Input: part model. Units: mm. Frame: model coordinates. A direction names the side the tool comes from. Give positions to 0.01 mm unless a question says otherwise; leave off trailing zeros. Loops run counter-clockwise (first coordinate to the right, second up) from the corner with the lowest first, then second, coordinate; pieces in that order, holes last. Notation, with made-up numbers: M 35.5,58 L 94.5,58 A28 ccw 94.5,90 Z; hole C 2.5,-38.75 d1. An arc over 180 degrees is marked long. One line per item, written item: value. Start each with the question number.
(1) Pin query (flat end, axial travel): P1, Ø0.6, axis at y = 11.5, z = -21.5, coming from the -X side; P2, Ø4.5, axis at x = -13.5, y = 11.5, coming from the +Z side; P3, Ø10.5, axis at x = -23.5, y = 18, coming from the -Z side; P4, Ø5, axis at x = -2, y = 13.5, coming from the +Z side. Return the tip coordinate at first contact, or that it passes through.
(2) Ray query, line 1 along X through (y, z) = (10.5, 61); line 2 along Z through (x, y) = (-23, 13.5); line 3 along X through (y, z) = (20, -17). Return the intervals inside material, ascending. Write a range as from..to.
(3) Section A-A on z = 50. Output: boundary loops of the cut face in (x, y), plus the area to 3 significant figures.
(4) Section B-B on z = 25.5. Output: boundary loops of the cut face in (x, y), plus the area to 3 significant figures.
(5) Pull-direction query (Z, two-part tool) for faces 1 (the flat face through (0, 9, -72.5)), 2 (the flat face through (-25, 25, -2.5)), 3 (the flat face through (8, 36, 37)), 4 (the flat face through (20.249, 11, -52)); classes: released by +Z, released by -Z, zero draft, split by the parting line, or undercut.
(6) Section C-C on z = -24.5. Output: boundary loops of the cut face in (x, y), plus the area to 3 significant figures.
(7) Access query for faces 5 (the flat face through (6.87, 7.48, -32.08)), 6 (the flat face through (-20.25, 30, -23)), 7 (the flat face through (7, 36, 63)), 8 (the flat face through (-3.75, 16, -32)). Directions: +Z, -Z, +X, -X, +Y, -Y. A direction counts if a zero-diameter tool reaches every point of the face in a straight line with its end or side. Return the directions, or none.
```python
from build123d import *

# Parameters (mm, degrees)
SKETCH_1_W                = 100
SKETCH_1_H                = 185
EXTRUDE_1_DEPTH           = 100
SKETCH_2_W                = 100
SKETCH_2_H                = 3.8
CUT_EXTRUDE_1_DEPTH       = 155
CUT_EXTRUDE_2_DEPTH       = 155
SKETCH_4_W                = 25.5
SKETCH_4_H                = 25.5
CUT_EXTRUDE_3_DEPTH       = 79
SKETCH_6_W                = 89.706259743
SKETCH_6_H                = 10
SKETCH_6_W_2              = 10.293740257
CUT_EXTRUDE_4_DEPTH       = 146.107718609
CUT_EXTRUDE_5_DEPTH       = 169.985946161
CUT_EXTRUDE_5_DEPTH_BACK  = 169.985946161
SKETCH_7_W                = 20
SKETCH_7_H                = 3.8
EXTRUDE_4_DEPTH           = 160
SKETCH_10_W               = 16
SKETCH_10_H               = 1.8
CUT_EXTRUDE_6_DEPTH       = 155
SKETCH_13_W               = 20
SKETCH_13_H               = 175
CUT_EXTRUDE_7_DEPTH       = 143.515578096
SKETCH_14_W               = 175
SKETCH_14_H               = 50
CUT_EXTRUDE_8_DEPTH       = 149.849756466
SKETCH_15_W               = 60
SKETCH_15_H               = 10
CUT_EXTRUDE_9_DEPTH       = 108.660066877
SKETCH_16_W               = 60
SKETCH_16_H               = 14.5
CUT_EXTRUDE_10_DEPTH      = 108.660066877
CUT_EXTRUDE_11_DEPTH      = 111.381157812
CUT_EXTRUDE_21_DEPTH      = 162.400898529
CUT_EXTRUDE_21_DEPTH_BACK = 140.5
CUT_EXTRUDE_26_DEPTH      = 111.381157983
SKETCH_34_W               = 10
SKETCH_34_H               = 20
CUT_EXTRUDE_31_DEPTH      = 96.490523251
SKETCH_35_W               = 18.74373947
SKETCH_35_H               = 80.5
CUT_EXTRUDE_32_DEPTH      = 14
CUT_EXTRUDE_35_DEPTH      = 60
CUT_EXTRUDE_36_DEPTH      = 140.5
SKETCH_43_W               = 0.25
SKETCH_43_H               = 0.002112168
CUT_EXTRUDE_37_DEPTH      = 140.5
SKETCH_44_W               = 7.5
SKETCH_44_H               = 0.502112168
CUT_EXTRUDE_38_DEPTH      = 80.4999
SKETCH_45_W               = 9.75
SKETCH_45_H               = 20
SKETCH_45_W_2             = 9.75146362
CUT_EXTRUDE_39_DEPTH      = 96.490523251
SKETCH_46_W               = 0.24853638
SKETCH_46_H               = 20
SKETCH_46_W_2             = 0.25
EXTRUDE_5_DEPTH           = 31.697888
CUT_EXTRUDE_40_DEPTH      = 106.399537724
CUT_EXTRUDE_40_DEPTH_BACK = 106.399537724
SKETCH_54_W               = 25.5
SKETCH_54_H               = 0.5
CUT_EXTRUDE_41_DEPTH      = 29


with BuildPart() as part:
    # 草图1 → 凸台-拉伸1 (new body)
    with BuildSketch(Plane(origin=(0, 0, 0), x_dir=(1, 0, 0), z_dir=(0, 1, 0))):
        Rectangle(SKETCH_1_W, SKETCH_1_H)
    extrude(amount=EXTRUDE_1_DEPTH)

    # 草图2 → 切除-拉伸1 (cut)
    with BuildSketch(Plane.XY.offset(92.5)):
        with Locations((0, 1.9)):
            Rectangle(SKETCH_2_W, SKETCH_2_H)
    extrude(amount=-CUT_EXTRUDE_1_DEPTH, mode=Mode.SUBTRACT)

    # 草图3 → 切除-拉伸2 (cut)
    with BuildSketch(Plane.XY.offset(92.5)):
        with BuildLine():
            Line((-20, 3.8), (-3.51, 3.8))
            ThreePointArc((-3.51, 3.8), (-3.949598778, 3.901619975), (-4.3, 4.185860522))
            Line((-4.3, 4.185860522), (-9.371869735, 10.69267521))
            ThreePointArc((-9.371869735, 10.69267521), (-9.267749528, 11.143089764), (-8.9765156, 11.502112168))
            Line((-8.9765156, 11.502112168), (-4.5, 11.502112168))
            ThreePointArc((-4.5, 11.502112168), (-4.146446609, 11.648558777), (-4, 12.002112168))
            Line((-4, 12.002112168), (-4, 16.002112168))
            Line((-4, 16.002112168), (-20, 16.002112168))
            Line((-20, 16.002112168), (-20, 3.8))
        make_face()
        with BuildLine():
            ThreePointArc((4.3, 4.185860522), (3.949598778, 3.901619975), (3.51, 3.8))
            Line((3.51, 3.8), (20, 3.8))
            Line((20, 3.8), (20, 16.002112168))
            Line((20, 16.002112168), (4, 16.002112168))
            Line((4, 16.002112168), (4, 12.002112168))
            ThreePointArc((4, 12.002112168), (4.146446609, 11.648558777), (4.5, 11.502112168))
            Line((4.5, 11.502112168), (8.9765156, 11.502112168))
            ThreePointArc((8.9765156, 11.502112168), (9.426930154, 11.220838522), (9.371869735, 10.69267521))
            Line((9.371869735, 10.69267521), (4.3, 4.185860522))
        make_face()
    extrude(amount=-CUT_EXTRUDE_2_DEPTH, mode=Mode.SUBTRACT)

    # 草图4 → 切除-拉伸3 (cut)
    with BuildSketch(Plane(origin=(0, 100, 0), x_dir=(1, 0, 0), z_dir=(0, 1, 0))):
        with Locations((7.75, -50.25)):
            Rectangle(SKETCH_4_W, SKETCH_4_H)
    extrude(amount=-CUT_EXTRUDE_3_DEPTH, mode=Mode.SUBTRACT)

    # 草图6 → 切除-拉伸4 (cut, through all)
    with BuildSketch(Plane(origin=(0, 100, 0), x_dir=(1, 0, 0), z_dir=(0, 1, 0))):
        with Locations((5.146870128, 87.5)):
            Rectangle(SKETCH_6_W, SKETCH_6_H)
        with Locations((-44.853129872, 87.5)):
            Rectangle(SKETCH_6_W_2, SKETCH_6_H)
    extrude(amount=-CUT_EXTRUDE_4_DEPTH, mode=Mode.SUBTRACT)

    # 草图7 → 切除-拉伸5 (cut, two sides: drawn at the far end of the back side and taken through both)
    with BuildSketch(Plane.ZY.offset(50).offset(-CUT_EXTRUDE_5_DEPTH_BACK)):
        with Locations((-72.5, 1.9)):
            Rectangle(SKETCH_7_W, SKETCH_7_H)
    extrude(amount=CUT_EXTRUDE_5_DEPTH + CUT_EXTRUDE_5_DEPTH_BACK, mode=Mode.SUBTRACT)

    # 草图9 → 凸台-拉伸4 (add)
    with BuildSketch(Plane.XY.offset(92.5)):
        Polygon((-9.371869735, 10.69267521), (-9.371869735, 13.29267521), (-4, 13.29267521), (4, 13.29267521), (9.371869735, 13.29267521), (9.371869735, 10.69267521), align=None)
    extrude(amount=-EXTRUDE_4_DEPTH)

    # 草图10 → 切除-拉伸6 (cut)
    with BuildSketch(Plane.XY.offset(92.5)):
        with Locations((-12, 16.902112168)):
            Rectangle(SKETCH_10_W, SKETCH_10_H)
        Polygon((4, 16.002112168), (4, 17.802112168), (19.99853638, 17.802112168), (20, 16.002112168), align=None)
    extrude(amount=-CUT_EXTRUDE_6_DEPTH, mode=Mode.SUBTRACT)

    # 草图13 → 切除-拉伸7 (cut, through all)
    with BuildSketch(Plane.XZ.offset(-3.8)):
        with Locations((-40, 5)):
            Rectangle(SKETCH_13_W, SKETCH_13_H)
        with Locations((40, 5)):
            Rectangle(SKETCH_13_W, SKETCH_13_H)
    extrude(amount=-CUT_EXTRUDE_7_DEPTH, mode=Mode.SUBTRACT)

    # 草图14 → 切除-拉伸8 (cut, through all)
    with BuildSketch(Plane(origin=(30, 0, 0), x_dir=(0, 0, -1), z_dir=(1, 0, 0))):
        with Locations((-5, 75)):
            Rectangle(SKETCH_14_W, SKETCH_14_H)
    extrude(amount=-CUT_EXTRUDE_8_DEPTH, mode=Mode.SUBTRACT)

    # 草图15 → 切除-拉伸9 (cut, through all)
    with BuildSketch(Plane.XZ.offset(-3.8)):
        with Locations((0, -77.5)):
            Rectangle(SKETCH_15_W, SKETCH_15_H)
    extrude(amount=-CUT_EXTRUDE_9_DEPTH, mode=Mode.SUBTRACT)

    # 草图16 → 切除-拉伸10 (cut, through all)
    with BuildSketch(Plane(origin=(0, 50, 0), x_dir=(1, 0, 0), z_dir=(0, 1, 0))):
        with Locations((0, -85.25)):
            Rectangle(SKETCH_16_W, SKETCH_16_H)
    extrude(amount=-CUT_EXTRUDE_10_DEPTH, mode=Mode.SUBTRACT)

    # 草图17 → 切除-拉伸11 (cut, through all)
    with BuildSketch(Plane(origin=(30, 0, 0), x_dir=(0, 0, -1), z_dir=(1, 0, 0))):
        with BuildLine():
            Line((72.5, 50), (-22.5, 50))
            add(Edge.make_bspline(
                [(-22.5, 50), (-9.330669895, 49.706144403), (11.085821801, 46.827148239), (38.239751221, 39.498978447), (59.688603115, 33.272875951), (70.679662454, 22.295526596), (72.5, 15.311284203)],
                knots=[0, 0, 0, 0, 0.374533404, 0.581855131, 0.802431491, 1, 1, 1, 1], degree=3))
            Line((72.5, 15.311284203), (72.5, 50))
        make_face()
    extrude(amount=-CUT_EXTRUDE_11_DEPTH, mode=Mode.SUBTRACT)

    # 草图24 → 切除-拉伸21 (cut, two sides: drawn at the far end of the back side and taken through both)
    with BuildSketch(Plane.XY.offset(78).offset(-CUT_EXTRUDE_21_DEPTH_BACK)):
        with BuildLine():
            Line((9.371869735, 11.309008937), (9.371869735, 10.69267521))
            ThreePointArc((9.371869735, 10.69267521), (9.477785695, 11.000842073), (9.371869735, 11.309008937))
        make_face()
    extrude(amount=CUT_EXTRUDE_21_DEPTH + CUT_EXTRUDE_21_DEPTH_BACK, mode=Mode.SUBTRACT)

    # 草图28 → 切除-拉伸26 (cut, through all)
    with BuildSketch(Plane(origin=(30, 0, 0), x_dir=(0, 0, -1), z_dir=(1, 0, 0))):
        with BuildLine():
            Line((-70.5, 50), (-78, 50))
            Line((-78, 50), (-78, 31.982866201))
            add(Edge.make_bspline(
                [(-70.5, 50), (-78.410932033, 48.656434308), (-77.0737544, 36.843285786), (-78, 31.982866201)],
                knots=[0, 0, 0, 0, 1, 1, 1, 1], degree=3))
        make_face()
    extrude(amount=-CUT_EXTRUDE_26_DEPTH, mode=Mode.SUBTRACT)

    # 草图34 → 切除-拉伸31 (cut, through all)
    with BuildSketch(Plane.XZ.offset(-3.8)):
        with Locations((-25, -32.5)):
            Rectangle(SKETCH_34_W, SKETCH_34_H)
        with Locations((25, -32.5)):
            Rectangle(SKETCH_34_W, SKETCH_34_H)
    extrude(amount=-CUT_EXTRUDE_31_DEPTH, mode=Mode.SUBTRACT)

    # 草图35 → 切除-拉伸32 (cut)
    with BuildSketch(Plane.XZ.offset(-3.8)):
        with Locations((0, 37.75)):
            Rectangle(SKETCH_35_W, SKETCH_35_H)
    extrude(amount=-CUT_EXTRUDE_32_DEPTH, mode=Mode.SUBTRACT)

    # 草图40 → 切除-拉伸35 (cut)
    with BuildSketch(Plane.XY.offset(-2.5)):
        Polygon((4, 13.29267521), (4, 17.8), (3.75, 17.8), (3.75, 12.79267521), (9.371869735, 12.79267521), (9.371869735, 13.29267521), align=None)
        Polygon((-3.75, 17.8), (-4, 17.8), (-4, 13.29267521), (-9.371869735, 13.29267521), (-9.371869735, 12.79267521), (-3.75, 12.79267521), align=None)
    extrude(amount=-CUT_EXTRUDE_35_DEPTH, mode=Mode.SUBTRACT)

    # 草图41 → 切除-拉伸36 (cut)
    with BuildSketch(Plane.XY.offset(78)):
        Polygon((-3.75, 18.302112168), (-20.25, 18.302112168), (-20.25, 3.8), (-20, 3.8), (-20, 17.802112168), (-3.75, 17.802112168), align=None)
        Polygon((3.75, 18.302112168), (3.75, 17.802112168), (19.99853638, 17.802112168), (19.99853638, 3.8), (20.24853638, 3.8), (20.24853638, 18.302112168), align=None)
    extrude(amount=-CUT_EXTRUDE_36_DEPTH, mode=Mode.SUBTRACT)

    # 草图43 → 切除-拉伸37 (cut)
    with BuildSketch(Plane.XY.offset(78)):
        with Locations((-3.875, 17.801056084)):
            Rectangle(SKETCH_43_W, SKETCH_43_H)
        with Locations((3.875, 17.801056084)):
            Rectangle(SKETCH_43_W, SKETCH_43_H)
    extrude(amount=-CUT_EXTRUDE_37_DEPTH, mode=Mode.SUBTRACT)

    # 草图44 → 切除-拉伸38 (cut)
    with BuildSketch(Plane.XY.offset(78)):
        with Locations((0, 18.051056084)):
            Rectangle(SKETCH_44_W, SKETCH_44_H)
    extrude(amount=-CUT_EXTRUDE_38_DEPTH, mode=Mode.SUBTRACT)

    # 草图45 → 切除-拉伸39 (cut, through all)
    with BuildSketch(Plane.XZ.offset(-3.8)):
        with Locations((-25.125, -12.5)):
            Rectangle(SKETCH_45_W, SKETCH_45_H)
        with Locations((25.12426819, -12.5)):
            Rectangle(SKETCH_45_W_2, SKETCH_45_H)
    extrude(amount=-CUT_EXTRUDE_39_DEPTH, mode=Mode.SUBTRACT)

    # 草图46 → 凸台-拉伸5 (add, through all)
    with BuildSketch(Plane.XZ.offset(-18.302112168)):
        with Locations((20.12426819, -32.5)):
            Rectangle(SKETCH_46_W, SKETCH_46_H)
        with Locations((-20.125, -32.5)):
            Rectangle(SKETCH_46_W_2, SKETCH_46_H)
    extrude(amount=-EXTRUDE_5_DEPTH)

    # 草图47 → 切除-拉伸40 (cut, two sides: drawn at the far end of the back side and taken through both)
    with BuildSketch(Plane.ZY.offset(20.25).offset(-CUT_EXTRUDE_40_DEPTH_BACK)):
        Polygon((-42.5, 38.203961841), (-22.5, 43.618048783), (-22.5, 50), (-42.5, 50), align=None)
    extrude(amount=CUT_EXTRUDE_40_DEPTH + CUT_EXTRUDE_40_DEPTH_BACK, mode=Mode.SUBTRACT)

    # 草图54 → 切除-拉伸41 (cut)
    with BuildSketch(Plane(origin=(0, 50, 0), x_dir=(1, 0, 0), z_dir=(0, 1, 0))):
        with Locations((7.75, -37.25)):
            Rectangle(SKETCH_54_W, SKETCH_54_H)
        Polygon((-5, -63), (-5, -37.5), (-5, -37), (-5.5, -37), (-5.5, -63), align=None)
    extrude(amount=-CUT_EXTRUDE_41_DEPTH, mode=Mode.SUBTRACT)


solid = part.part
```
Output values:
1. P1: stops at x = -9.37
1. P2: stops at z = -62.5
1. P3: stops at z = -72.5
1. P4: stops at z = -2.5
2. line 1: x = -30..-20.25, 20.25..30
2. line 2: z = -72.5..-42.5, -2.5..78
2. line 3: x = -20.25..20.25
3. outline: M -30,3.8 L -20.25,3.8 L -20.25,18.3 L 20.25,18.3 L 20.25,3.8 L 30,3.8 L 30,50 L 20.5,50 L 20.5,21 L -5.5,21 L -5.5,50 L -30,50 Z
3. area: 1,430 mm²
4. outline: M -30,3.8 L -20.25,3.8 L -20.25,18.3 L 20.25,18.3 L 20.25,3.8 L 30,3.8 L 30,50 L -30,50 Z
4. area: 2,180 mm²
5. face 1: released by -Z
5. face 2: undercut
5. face 3: undercut
5. face 4: zero draft
6. outline: M -20.25,18.3 L -3.75,18.3 L -3.75,12.79 L -9.37,12.79 L -9.37,10.69 L -4.3,4.19 A1 ccw -3.51,3.8 L 3.51,3.8 A1 ccw 4.3,4.19 L 9.37,10.69 L 9.37,12.79 L 3.75,12.79 L 3.75,18.3 L 20.25,18.3 L 20.25,43.08 L -20.25,43.08 Z
6. area: 1,180 mm²
7. face 5: +Z, -Y
7. face 6: -X, +Y, -Y
7. face 7: +Y
7. face 8: +Z
